Here's how the part is built. I have some questions about the finished solid (model axes, mm). A direction names the side the tool comes from. Coordinates: 2 decimals unless noted, no trailing zeros. Order: outer loops, then holes, each group sorted by start corner. A loop starts at its lowest first (then second) coordinate and runs counter-clockwise, first axis right, second up. Notation, with made-up numbers: (-15.75, -16) - (34.25, -16) arc R17 cw to (34.25, -12) - close; hole circle Ø1 at (-20, 1.5). An arc over 180 degrees is marked (long way). Answer in a Markdown table with one row per item. Add a question column.
Item 1: I want a section at A-A (y = 0). Please give me the cut outline in (x, z) (3 decimals), plus the area to 3 significant figures.
Item 2: I want a section at B-B (x = 0). Please give me the cut outline in (y, z) (3 decimals).
Item 3: If I drill on line 1 along Y through (x, z) = (0, -2.75) (3 decimals); line 2 along Z through (x, y) = (14, 11); line 3 along Y through (x, z) = (-4, 2.5), over which ranges is the centre line in solid material (lowest first)? Write a range as from..to.
Item 4: I want a section at C-C (z = -2.75). Please give me the cut outline in (x, y) (3 decimals).
Item 5: Will these pins go through, and if not, where does the flat tip stop? pin 1 Ø5 at (x, z) = (-1, 0.5) entering from -Y; pin 2 Ø5 at (x, y) = (0, 0) entering from -Z; pin 3 Ø5 at (x, z) = (-5, 0) entering from -Y.
Item 6: I want a section at D-D (z = 8.5). Please give me the cut outline in (x, y) (3 decimals), plus the area to 3 significant figures.
Item 7: On a 3-axis mill with a long thin cutter (end or side, diameter ignored), from which of +Z, -Z, +X, -X, +Y, -Y can I reach the whole of each face in a straight line? I mean faces 1 (the cylindrical face through (0.69, 3.1, -3.13)), 2 (the flat face through (0, -4, -6.35)), 3 (the cylindrical face through (-0.69, 15.8, 9.48)). Say none if no direction works.
Item 8: Thinking about a two-plate mould opening in Y: for faces 4 (the cylindrical face through (-3.9, 7.6, -3.1)), 5 (the flat face through (0, 0, 0)), 6 (the flat face through (0, 13, 12.7)), which applies, +Y half, -Y half, draft (parallel to the pull), parting line (faces both ways), or undercut?
Autodesk Inventor part; units mm, degrees
ref_plane "XZ Plane" through (0, 0, 0) normal (0, 1, 0) x (-1, 0, 0)
ref_plane "XY Plane" through (0, 0, 0) normal (0, 0, 1) x (1, 0, 0)
sketch "Sketch1" plane through (0, 0, 0) normal (0, 0, 1) x (1, 0, 0)
  circle A0 centre (0, 0) radius 21.7258
extrude "Extrusion1" add sketch "Sketch1" along normal blind 6.35
sketch "Sketch2" plane through (0, 0, 6.35) normal (0, 0, 1) x (1, 0, 0)
  circle A0 centre (0, 12.7) radius 3.175
  point P0 (0, 0)
  dimension "d4" = 6.35
extrude "Extrusion2" add sketch "Sketch2" along normal blind 6.35
sketch "Sketch5" plane through (0, 0, 0) normal (0, 0, -1) x (-1, 0, 0)
  circle A0 centre (0, 0) radius 3.175
  circle A1 centre (0, 0) radius 8.542
  point P0 (0, 0)
ref_plane "Work Plane3" through (0, 0, -6.35) normal (0, 0, -1) x (-1, 0, 0)
extrude "Extrusion5" add sketch "Sketch5" along normal blind 6.35
sketch "Sketch6" plane through (0, 0, -6.35) normal (0, 0, -1) x (-1, 0, 0)
  circle A0 centre (0, 0) radius 3.175
  spline S0 degree 4 poles (-15.875, 0) (-15.875, 5.123) (-15.6795, 13.2839) (0.7771, 27.615) (13.6923, 12.2077) (15.875, 5.0189) (15.875, 0) knots -1 -1 -1 -1 -1 -0.623021 -0.373021 0 0 0 0 0
  spline S1 degree 4 poles (15.875, 0) (15.875, -4.6644) (10.9112, -18.4609) (-6.6696, -14.611) (-16.1915, -10.8158) (-15.875, 0) knots -1 -1 -1 -1 -1 -0.624992 0 0 0 0 0
  point P0 (0, 0)
extrude "Extrusion4" [suppressed]
sketch "Sketch7" plane through (0, 0, -12.7) normal (0, 0, -1) x (-1, 0, 0)
  circle A0 centre (0, 0) radius 3.175
  point P0 (0, 0)
  point P1 (15.875, 0)
  point P2 (-15.875, 0)
properties part number "Eccentric" material "Steel"
Values follow:
| question | item | result |
|---|---|---|
| 1 | outline | (-21.726, 0) - (-8.542, 0) - (-8.542, -6.35) - (-3.175, -6.35) - (-3.175, 0) - (3.175, 0) - (3.175, -6.35) - (8.542, -6.35) - (8.542, 0) - (21.726, 0) - (21.726, 6.35) - (-21.726, 6.35) - close |
| 1 | area | 344 mm^2 |
| 2 | outline | (-21.726, 0) - (-8.542, 0) - (-8.542, -6.35) - (-3.175, -6.35) - (-3.175, 0) - (3.175, 0) - (3.175, -6.35) - (8.542, -6.35) - (8.542, 0) - (21.726, 0) - (21.726, 6.35) - (15.875, 6.35) - (15.875, 12.7) - (9.525, 12.7) - (9.525, 6.35) - (-21.726, 6.35) - close |
| 3 | line 1 | y = -8.542..-3.175, 3.175..8.542 |
| 3 | line 2 | z = 0..6.35 |
| 3 | line 3 | y = -21.35..21.35 |
| 4 | outline | circle Ø17.084 at (0, 0); hole circle Ø6.35 at (0, 0) |
| 5 | pin 1 | stops at y = -21.73 |
| 5 | pin 2 | stops at z = 0 |
| 5 | pin 3 | stops at y = -21.58 |
| 6 | outline | circle Ø6.35 at (0, 12.7) |
| 6 | area | 31.7 mm^2 |
| 7 | face 1 | -Z |
| 7 | face 2 | -Z, +X, -X, +Y, -Y |
| 7 | face 3 | +Z |
| 8 | face 4 | parting line |
| 8 | face 5 | undercut |
| 8 | face 6 | draft |
